Could you check a few things on this model? Use its own coordinates, in mm. A direction names the side the tool comes from. Give positions to 0.01 mm unless a question says otherwise; leave off trailing zeros. Loops run counter-clockwise (first coordinate to the right, second up) from the corner with the lowest first, then second, coordinate; pieces in that order, holes last. Notation, with made-up numbers: (85, 15) - (117, 15) arc R28 ccw to (117, 34) - close; hole circle Ø4 at (16.5, 40.5). An arc over 180 degrees is marked (long way). Write each question's results on one line, items separated by ' | '. Start each with the question number.
```python
from build123d import *

# Parameters (mm, degrees)
SZKIC1_R                    = 2.6
SZKIC1_R_2                  = 1.55
DODANIE_WYCI_GNI_CIE1_DEPTH = 2.5
SZKIC2_R                    = 1.55
DODANIE_WYCI_GNI_CIE2_DEPTH = 1


with BuildPart() as part:
    # Szkic1 → Dodanie-wyciągnięcie1 (new body)
    with BuildSketch(Plane.XY):
        Circle(SZKIC1_R)
        Circle(SZKIC1_R_2, mode=Mode.SUBTRACT)
    extrude(amount=DODANIE_WYCI_GNI_CIE1_DEPTH)

    # Szkic2 → Dodanie-wyciągnięcie2 (add)
    with BuildSketch(Plane.XY.offset(2.5)):
        with BuildLine():
            Line((-2.6, -1), (-2.6, 1))
            ThreePointArc((-2.6, 1), (0, 3.6), (2.6, 1))
            Line((2.6, 1), (2.6, -1))
            ThreePointArc((2.6, -1), (0, -3.6), (-2.6, -1))
        make_face()
        Circle(SZKIC2_R, mode=Mode.SUBTRACT)
    extrude(amount=DODANIE_WYCI_GNI_CIE2_DEPTH)


solid = part.part
```
Q1. I'm going to push flat-ended pins straight in: pin 1 Ø1.9 at (x, y) = (0, 0) entering from -Z; pin 2 Ø3 at (x, y) = (0.5, -2) entering from -Z. Where does each tip first touch, or does it pass through?
Q2. I want a section at D-D, the plane x = 0.75. List the corners of the cut face in (y, z) for me, then the cut area to 3 significant figures.
Q3. I need wall thicknesses on L1, parallel to Y at x = 0, z = 0.95; L2, parallel to X at y = 1, z = 0.9. Which ranges of each line are inside material? Lowest first, please. Write a range as from..to.
Q4. I want a section at C-C, the plane y = 2. List the corners of the cut face in (x, z) for me.
Q5. I want a section at B-B, the plane z = 3.15. List the corners of the cut face in (x, y) for me, then the cut area to 3 significant figures.
Q6. Which directions (+Z, -Z, +X, -X, +Y, -Y) give clear straight access to the entire face, cutting with the end or side of a thin tool? Please do faces 1 (the face through (0, 3, 2.5)), 2 (the face through (-0.338, 2.578, 1.232)), 3 (the face through (-2.6, 0, 3)).
Q7. I want a section at A-A, the plane x = 0. List the corners of the cut face in (y, z) for me, then the cut area to 3 significant figures.
Q8. If we mould it in two halves opening along X, with no side actions, what happens to faces 4 (the face through (0.715, -1.375, 1.726)), 5 (the face through (2.6, 0, 3)), 6 (the face through (0, -3, 2.5))? For each: +X half, -X half, draft (parallel to the pull), parting line (faces both ways), or undercut.
Conclusion:
1) pin 1: through | pin 2: z = 0
2) outline: (-3.49, 2.5) - (-2.49, 2.5) - (-2.49, 0) - (-1.36, 0) - (-1.36, 3.5) - (-3.49, 3.5) - close; (1.36, 0) - (2.49, 0) - (2.49, 2.5) - (3.49, 2.5) - (3.49, 3.5) - (1.36, 3.5) - close | area: 9.93 mm^2
3) L1: -2.6..-1.55, 1.55..2.6 | L2: -2.4..-1.18, 1.18..2.4
4) outline: (-2.4, 2.5) - (-1.66, 2.5) - (-1.66, 0) - (1.66, 0) - (1.66, 2.5) - (2.4, 2.5) - (2.4, 3.5) - (-2.4, 3.5) - close
5) outline: (-2.6, -1) arc R2.6 ccw to (2.6, -1) - (2.6, 1) arc R2.6 ccw to (-2.6, 1) - close; hole circle Ø3.1 at (0, 0) | area: 24.1 mm^2
6) face 1: -Z, +Y | face 2: -Z | face 3: +Z, -Z, -X, +Y, -Y
7) outline: (-3.6, 2.5) - (-2.6, 2.5) - (-2.6, 0) - (-1.55, 0) - (-1.55, 3.5) - (-3.6, 3.5) - close; (1.55, 0) - (2.6, 0) - (2.6, 2.5) - (3.6, 2.5) - (3.6, 3.5) - (1.55, 3.5) - close | area: 9.35 mm^2
8) face 4: undercut | face 5: +X half | face 6: draft
